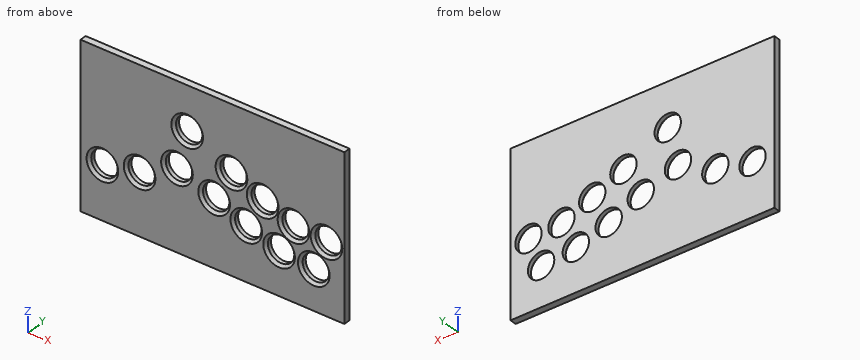
```python
from build123d import *

# Parameters (mm, degrees)
SKETCH1_W           = 200
SKETCH1_H           = 123.6
SKETCH1_R           = 10
BOSS_EXTRUDE1_DEPTH = 5
CHAMFER1_SIZE       = 2


with BuildPart() as part:
    # Sketch1 → Boss-Extrude1 (new body)
    with BuildSketch(Plane(origin=(0, 0, 0), x_dir=(1, 0, 0), z_dir=(0, 1, 0))):
        with Locations((-11.382571905, -37.613815878)):
            Rectangle(SKETCH1_W, SKETCH1_H)
        with Locations(Location((-30.546222192, -66.351509684, 0), (0, 0, 270))):
            Circle(SKETCH1_R, mode=Mode.SUBTRACT)
        with Locations(Location((-66.632534539, -22.057178609, 0), (0, 0, 270))):
            Circle(SKETCH1_R, mode=Mode.SUBTRACT)
        with Locations(Location((-94.823650655, -15.979370187, 0), (0, 0, 270))):
            Circle(SKETCH1_R, mode=Mode.SUBTRACT)
        with Locations(Location((-10.090347172, -26.425303761, 0), (0, 0, 270))):
            Circle(SKETCH1_R, mode=Mode.SUBTRACT)
        with Locations(Location((65.449469323, -6.002101711, 0), (0, 0, 270))):
            Circle(SKETCH1_R, mode=Mode.SUBTRACT)
        with Locations(Location((39.120524561, -8.47636758, 0), (0, 0, 270))):
            Circle(SKETCH1_R, mode=Mode.SUBTRACT)
        with Locations(Location((3.050131898, -49.923740932, 0), (0, 0, 270))):
            Circle(SKETCH1_R, mode=Mode.SUBTRACT)
        with Locations(Location((26.684644812, -39.329734959, 0), (0, 0, 270))):
            Circle(SKETCH1_R, mode=Mode.SUBTRACT)
        with Locations(Location((50.034895937, -30.657694114, 0), (0, 0, 270))):
            Circle(SKETCH1_R, mode=Mode.SUBTRACT)
        with Locations(Location((-38.286901535, -36.422907606, 0), (0, 0, 270))):
            Circle(SKETCH1_R, mode=Mode.SUBTRACT)
        with Locations(Location((75.040753418, -29.205017129, 0), (0, 0, 270))):
            Circle(SKETCH1_R, mode=Mode.SUBTRACT)
        with Locations(Location((14.228770638, -16.291965116, 0), (0, 0, 270))):
            Circle(SKETCH1_R, mode=Mode.SUBTRACT)
    extrude(amount=BOSS_EXTRUDE1_DEPTH)

    # Chamfer1
    chamfer1_edges = [part.edges().sort_by_distance(p)[0] for p in [
        (-30.546222192, 0, 56.351509684),
        (-66.632534539, 0, 12.057178609),
        (-94.823650655, 0, 5.979370187),
        (-10.090347172, 0, 16.425303761),
        (65.449469323, 0, -3.997898289),
        (39.120524561, 0, -1.52363242),
        (3.050131898, 0, 39.923740932),
        (26.684644812, 0, 29.329734959),
        (50.034895937, 0, 20.657694114),
        (-38.286901535, 0, 26.422907606),
        (75.040753418, 0, 19.205017129),
        (14.228770638, 0, 6.291965116),
    ]]
    chamfer(chamfer1_edges, length=CHAMFER1_SIZE)


solid = part.part
```
Check sheet for the modelled part. Datum: model origin and axes. Units: mm. Give positions to 0.01 mm unless a question says otherwise; leave off trailing zeros. Answer as CSV lines item,"result".
Item 1: Scan lines: L1, parallel to X at y = 0.6, z = 36; L2, parallel to Z at x = 22.5, y = 2.2; L3, parallel to X at y = 3.7, z = 66. Record each from-to range of solid material in increasing order.
Reply:
L1,"-111.38 to -49.68, -26.89 to -16.28, -3.9 to 15.78, 37.59 to 39.96, 60.11 to 65.89, 84.19 to 88.62"
L2,"-24.19 to 10.67, 21.91 to 30.25, 48.41 to 99.41"
L3,"-111.38 to -40.54, -20.55 to 88.62"
Item 2: Depth check by flat-ended pin: pin 1 Ø12 at (x, z) = (3.05, 49.92) entering from +Y; pin 2 Ø23 at (x, z) = (-38.29, 36.42) entering from -Y. Enter the tip coordinate at first touch or a pass-through.
Reply:
pin 1,"through"
pin 2,"y = 0.5"
Item 3: Sectioned sample at A-A, the plane y = 4.15. State how many separate pieces and enclosed holes the cut face has, then the cut area to 3 significant figures.
Reply:
separate pieces,"1"
enclosed holes,"12"
area,"21,000 mm^2"
